from build123d import *

# Parameters (mm, degrees)
F0_R     = 47.625
F1_DEPTH = 1.5875
F0_R_2   = 50.8
F2_DEPTH = 25.4


with BuildPart() as f1:
    # F0 (on Top) → F1 (new body)
    with BuildSketch(Plane.XY):
        Circle(F0_R)
        with BuildLine():
            Line((-14.920541, -42.067761), (-6.444111, -15.979992))
            ThreePointArc((-6.444111, -15.979992), (-4.943836, -15.215563), (-4.179408, -16.715838))
            Line((-4.179408, -16.715838), (-12.655838, -42.803608))
            ThreePointArc((-12.655838, -42.803608), (-14.156113, -43.568036), (-14.920541, -42.067761))
        make_face(mode=Mode.SUBTRACT)
        with BuildLine():
            ThreePointArc((-1.190625, -7.540625), (0, -6.35), (1.190625, -7.540625))
            Line((1.190625, -7.540625), (1.190625, -43.894375))
            ThreePointArc((1.190625, -43.894375), (0, -45.085), (-1.190625, -43.894375))
            Line((-1.190625, -43.894375), (-1.190625, -7.540625))
        make_face(mode=Mode.SUBTRACT)
        with BuildLine():
            Line((-44.619519, 1.190625), (-17.189215, 1.190625))
            ThreePointArc((-17.189215, 1.190625), (-15.99859, 0), (-17.189215, -1.190625))
            Line((-17.189215, -1.190625), (-44.619519, -1.190625))
            ThreePointArc((-44.619519, -1.190625), (-45.810144, 0), (-44.619519, 1.190625))
        make_face(mode=Mode.SUBTRACT)
        with BuildLine():
            ThreePointArc((-5.395504, -5.400662), (-3.732436, -5.137258), (-3.469032, -6.800326))
            Line((-3.469032, -6.800326), (-24.83723, -36.211127))
            ThreePointArc((-24.83723, -36.211127), (-26.500298, -36.474531), (-26.763702, -34.811464))
            Line((-26.763702, -34.811464), (-5.395504, -5.400662))
        make_face(mode=Mode.SUBTRACT)
        with BuildLine():
            Line((-36.797781, -25.263459), (-14.606199, -9.140331))
            ThreePointArc((-14.606199, -9.140331), (-12.943131, -9.403735), (-13.206535, -11.066803))
            Line((-13.206535, -11.066803), (-35.398117, -27.189931))
            ThreePointArc((-35.398117, -27.189931), (-37.061185, -26.926527), (-36.797781, -25.263459))
        make_face(mode=Mode.SUBTRACT)
        with BuildLine():
            ThreePointArc((-7.539484, -1.19783), (-6.039209, -1.962258), (-6.803637, -3.462533))
            Line((-6.803637, -3.462533), (-41.378108, -14.696459))
            ThreePointArc((-41.378108, -14.696459), (-42.878383, -13.932031), (-42.113955, -12.431756))
            Line((-42.113955, -12.431756), (-7.539484, -1.19783))
        make_face(mode=Mode.SUBTRACT)
        with BuildLine():
            Line((12.655838, -42.803608), (4.179408, -16.715838))
            ThreePointArc((4.179408, -16.715838), (4.943836, -15.215563), (6.444111, -15.979992))
            Line((6.444111, -15.979992), (14.920541, -42.067761))
            ThreePointArc((14.920541, -42.067761), (14.156113, -43.568036), (12.655838, -42.803608))
        make_face(mode=Mode.SUBTRACT)
        with BuildLine():
            ThreePointArc((3.469032, -6.800326), (3.732436, -5.137258), (5.395504, -5.400662))
            Line((5.395504, -5.400662), (26.763702, -34.811464))
            ThreePointArc((26.763702, -34.811464), (26.500298, -36.474531), (24.83723, -36.211127))
            Line((24.83723, -36.211127), (3.469032, -6.800326))
        make_face(mode=Mode.SUBTRACT)
        with BuildLine():
            Line((35.398117, -27.189931), (13.206535, -11.066803))
            ThreePointArc((13.206535, -11.066803), (12.943131, -9.403735), (14.606199, -9.140331))
            Line((14.606199, -9.140331), (36.797781, -25.263459))
            ThreePointArc((36.797781, -25.263459), (37.061185, -26.926527), (35.398117, -27.189931))
        make_face(mode=Mode.SUBTRACT)
        with BuildLine():
            ThreePointArc((6.803637, -3.462533), (6.039209, -1.962258), (7.539484, -1.19783))
            Line((7.539484, -1.19783), (42.113955, -12.431756))
            ThreePointArc((42.113955, -12.431756), (42.878383, -13.932031), (41.378108, -14.696459))
            Line((41.378108, -14.696459), (6.803637, -3.462533))
        make_face(mode=Mode.SUBTRACT)
        with BuildLine():
            Line((44.619519, -1.190625), (17.189215, -1.190625))
            ThreePointArc((17.189215, -1.190625), (15.99859, 0), (17.189215, 1.190625))
            Line((17.189215, 1.190625), (44.619519, 1.190625))
            ThreePointArc((44.619519, 1.190625), (45.810144, 0), (44.619519, -1.190625))
        make_face(mode=Mode.SUBTRACT)
        with BuildLine():
            ThreePointArc((-6.803637, 3.462533), (-6.039209, 1.962258), (-7.539484, 1.19783))
            Line((-7.539484, 1.19783), (-42.113955, 12.431756))
            ThreePointArc((-42.113955, 12.431756), (-42.878383, 13.932031), (-41.378108, 14.696459))
            Line((-41.378108, 14.696459), (-6.803637, 3.462533))
        make_face(mode=Mode.SUBTRACT)
        with BuildLine():
            Line((-35.398117, 27.189931), (-13.206535, 11.066803))
            ThreePointArc((-13.206535, 11.066803), (-12.943131, 9.403735), (-14.606199, 9.140331))
            Line((-14.606199, 9.140331), (-36.797781, 25.263459))
            ThreePointArc((-36.797781, 25.263459), (-37.061185, 26.926527), (-35.398117, 27.189931))
        make_face(mode=Mode.SUBTRACT)
        with BuildLine():
            ThreePointArc((-3.469032, 6.800326), (-3.732436, 5.137258), (-5.395504, 5.400662))
            Line((-5.395504, 5.400662), (-26.763702, 34.811464))
            ThreePointArc((-26.763702, 34.811464), (-26.500298, 36.474531), (-24.83723, 36.211127))
            Line((-24.83723, 36.211127), (-3.469032, 6.800326))
        make_face(mode=Mode.SUBTRACT)
        with BuildLine():
            Line((-12.655838, 42.803608), (-4.179408, 16.715838))
            ThreePointArc((-4.179408, 16.715838), (-4.943836, 15.215563), (-6.444111, 15.979992))
            Line((-6.444111, 15.979992), (-14.920541, 42.067761))
            ThreePointArc((-14.920541, 42.067761), (-14.156113, 43.568036), (-12.655838, 42.803608))
        make_face(mode=Mode.SUBTRACT)
        with BuildLine():
            ThreePointArc((-1.190625, 43.894375), (0, 45.085), (1.190625, 43.894375))
            Line((1.190625, 43.894375), (1.190625, 7.540625))
            ThreePointArc((1.190625, 7.540625), (0, 6.35), (-1.190625, 7.540625))
            Line((-1.190625, 7.540625), (-1.190625, 43.894375))
        make_face(mode=Mode.SUBTRACT)
        with BuildLine():
            ThreePointArc((7.539484, 1.19783), (6.039209, 1.962258), (6.803637, 3.462533))
            Line((6.803637, 3.462533), (41.378108, 14.696459))
            ThreePointArc((41.378108, 14.696459), (42.878383, 13.932031), (42.113955, 12.431756))
            Line((42.113955, 12.431756), (7.539484, 1.19783))
        make_face(mode=Mode.SUBTRACT)
        with BuildLine():
            Line((36.797781, 25.263459), (14.606199, 9.140331))
            ThreePointArc((14.606199, 9.140331), (12.943131, 9.403735), (13.206535, 11.066803))
            Line((13.206535, 11.066803), (35.398117, 27.189931))
            ThreePointArc((35.398117, 27.189931), (37.061185, 26.926527), (36.797781, 25.263459))
        make_face(mode=Mode.SUBTRACT)
        with BuildLine():
            ThreePointArc((5.395504, 5.400662), (3.732436, 5.137258), (3.469032, 6.800326))
            Line((3.469032, 6.800326), (24.83723, 36.211127))
            ThreePointArc((24.83723, 36.211127), (26.500298, 36.474531), (26.763702, 34.811464))
            Line((26.763702, 34.811464), (5.395504, 5.400662))
        make_face(mode=Mode.SUBTRACT)
        with BuildLine():
            ThreePointArc((12.655838, 42.803608), (14.156113, 43.568036), (14.920541, 42.067761))
            Line((14.920541, 42.067761), (6.444111, 15.979992))
            ThreePointArc((6.444111, 15.979992), (4.943836, 15.215563), (4.179408, 16.715838))
            Line((4.179408, 16.715838), (12.655838, 42.803608))
        make_face(mode=Mode.SUBTRACT)
    extrude(amount=F1_DEPTH)

    # F0 (on Top) → F2 (join)
    with BuildSketch(Plane.XY):
        Circle(F0_R_2)
        Circle(F0_R, mode=Mode.SUBTRACT)
    extrude(amount=F2_DEPTH)


solid = f1.part
Model file for the job. Use its own axes, mm. A direction names the side the tool comes from. Round coordinates to 2 decimals unless told otherwise and drop trailing zeros. Order: outer loops, then holes, each group sorted by start corner. A loop starts at its lowest first (then second) coordinate and runs counter-clockwise, first axis right, second up.
(1) 3-axis set-ups, long thin cutter, end or side, ignore diameter. For faces 1 (the face through (-24.333, 9.158, 0.783)), 2 (the face through (-1, 1, 0)): which of +Z, -Z, +X, -X, +Y, -Y reach the whole face in a straight line?
(2) Drill centre lines: line 1 (Y direction, x = 0, z = 12.5) (3 decimals); line 2 (Y direction, x = 31, z = 1.5); line 3 (Z direction, x = 37.5, y = 28). Where is each one in solid material? Low to high.
(3) Band-saw the part on A-A (x = 0). Give the number of separate pieces and of enclosed holes in the cut face, then the cut area to 3 significant figures.
(4) Pin check, flat tips, straight feed: pin 1 (0.8 mm diameter, centred on y = 26, z = 1, fed in from +X); pin 2 (1.7 mm diameter, centred on y = 19, z = 1, fed in from -X); pin 3 (6 mm diameter, centred on x = 7.5, y = 4.5, fed in from -Z); pin 4 (6 mm diameter, centred on y = 18.5, z = 19.5, fed in from +X). Stop position of each tip, or through.
(5) Band-saw the part on B-B (x = 29). List the corners of the cut face in (y, z).
(6) Pull direction Y, two halves, no side cores. Call faces 3 (the face through (-25.857, -17.315, 0.783)), 4 (the face through (-15.3, 45.4, 25.4)): released by +Y, released by -Y, zero draft, split by the parting line, or undercut.
(7) Band-saw the part on C-C (z = 3). List the corners of the cut face in (x, y) (3 decimals).
Verdict:
1. face 1: +Z, -Z
1. face 2: -Z, +X, -X, +Y, -Y
2. line 1: y = -50.8 to -47.625, 47.625 to 50.8
2. line 2: y = -40.24 to -23.99, -21.05 to -11.32, -8.82 to -1.19, 1.19 to 8.82, 11.32 to 21.05, 23.99 to 40.24
2. line 3: z = 0 to 1.59
3. separate pieces: 3
3. enclosed holes: 0
3. area: 190 mm2
4. pin 1: stops at x = 43.88
4. pin 2: stops at x = -47.45
4. pin 3: stops at z = 0
4. pin 4: stops at x = 48.38
5. outline: (-41.71, 0) - (-22.54, 0) - (-22.54, 1.59) - (-37.78, 1.59) - (-37.78, 25.4) - (-41.71, 25.4) - close; (-19.6, 0) - (-10.67, 0) - (-10.67, 1.59) - (-19.6, 1.59) - close; (-8.17, 0) - (-1.19, 0) - (-1.19, 1.59) - (-8.17, 1.59) - close; (1.19, 0) - (8.17, 0) - (8.17, 1.59) - (1.19, 1.59) - close; (10.67, 0) - (19.6, 0) - (19.6, 1.59) - (10.67, 1.59) - close; (22.54, 0) - (41.71, 0) - (41.71, 25.4) - (37.78, 25.4) - (37.78, 1.59) - (22.54, 1.59) - close
6. face 3: undercut
6. face 4: zero draft
7. outline: circle Ø101.6 at (0, 0); hole circle Ø95.25 at (0, 0)
